Design review of the part built by this model. Coordinates are the model's own, in mm. A direction names the side the tool comes from. Coordinates: 2 decimals unless noted, no trailing zeros. Write each loop counter-clockwise with the first axis right and the second up, starting at its lowest first coordinate (ties: lowest second). Pieces come first, ordered by that corner, then holes. Notation, with made-up numbers: M 33.25,24 L 74.25,24 A26 cw 74.25,46 Z; hole C 19.5,63 d2. An arc over 180 degrees is marked long. Write each question's results on one line, items separated by ' | '. Start each with the question number.
```python
from build123d import *

# Parameters (mm, degrees)
F0_R     = 1.5
F1_DEPTH = 4


with BuildPart() as f1:
    # F0 (on Top) → F1 (new body)
    with BuildSketch(Plane.XY):
        with BuildLine():
            Line((10, 68.838424), (-25, 68.838424))
            Line((-25, 68.838424), (-25, 56.048434))
            Line((-25, 56.048434), (-15.945247, 35.027615))
            ThreePointArc((-15.945247, 35.027615), (-34.796929, 16.442581), (-37.185223, -9.921893))
            Line((-37.185223, -9.921893), (-47.426407, -15.834643))
            Line((-47.426407, -15.834643), (-56.234754, -20.920145))
            Line((-56.234754, -20.920145), (-64.615824, -25.758958))
            Line((-64.615824, -25.758958), (-47.115824, -56.069847))
            Line((-47.115824, -56.069847), (-36.039368, -49.674852))
            Line((-36.039368, -49.674852), (-29.243596, -40.556283))
            Line((-29.243596, -40.556283), (-22.362181, -31.322797))
            ThreePointArc((-22.362181, -31.322797), (3.158772, -38.356315), (27.185223, -27.242401))
            Line((27.185223, -27.242401), (37.426407, -33.155151))
            Line((37.426407, -33.155151), (46.234754, -38.240653))
            Line((46.234754, -38.240653), (54.615824, -43.079466))
            Line((54.615824, -43.079466), (72.115824, -12.768577))
            Line((72.115824, -12.768577), (61.039368, -6.373582))
            Line((61.039368, -6.373582), (49.744569, -5.047556))
            Line((49.744569, -5.047556), (38.307428, -3.704819))
            ThreePointArc((38.307428, -3.704819), (31.638157, 21.913734), (10, 37.164294))
            Line((10, 37.164294), (10, 59.160798))
            Line((10, 59.160798), (10, 68.838424))
        make_face()
        with Locations((-45.651723, -50.605746)):
            Circle(F0_R, mode=Mode.SUBTRACT)
        with Locations((-54.151723, -35.883314)):
            Circle(F0_R, mode=Mode.SUBTRACT)
        with Locations((-14.314554, -12.883314)):
            Circle(F0_R, mode=Mode.SUBTRACT)
        with Locations((58.151723, -28.955111)):
            Circle(F0_R, mode=Mode.SUBTRACT)
        with Locations((18.314554, -5.955111)):
            Circle(F0_R, mode=Mode.SUBTRACT)
        with Locations((66.651723, -14.232679)):
            Circle(F0_R, mode=Mode.SUBTRACT)
        with Locations((-4, 18.838424)):
            Circle(F0_R, mode=Mode.SUBTRACT)
        with Locations((-21, 64.838424)):
            Circle(F0_R, mode=Mode.SUBTRACT)
        with Locations((-4, 64.838424)):
            Circle(F0_R, mode=Mode.SUBTRACT)
    extrude(amount=F1_DEPTH)


solid = f1.part
```
Item 1: For faces 5 (the flat face through (-25, 63, 2)), 6 (the cylindrical face through (-12.93, -13.46, 1.97)), list the 3-axis set-ups (+Z, -Z, +X, -X, +Y, -Y) from which the entire face can be reached by the end or side of a thin tool; tool diameter is ignored.
Item 2: Draft analysis for pull direction X (two halves, no side actions). For faces 1 (the flat face through (3, -7, 0)), 2 (the cylindrical face through (58.96, -27.69, 1.97)), 3 (the flat face through (-20.54, 45.69, 1.97)), 4 (the flat face through (10, 53, 2)), state which applies: released by +X, released by -X, zero draft, split by the parting line, or undercut.
Item 3: We need section B-B on x = -4. State the section outline as (y, z) points, then the cut area to 3 significant figures.
Item 4: Wall thickness on L1, parallel to Y at x = -4, z = 2.8; L2, parallel to Y at x = -4.5, z = 0.5; L3, parallel to X at y = -50, z = 2.2: over which ranges is each line inside the solid? List them lowest first.
Item 5: We need section C-C on x = 44.5. State the section outline as (y, z) points, then the cut area to 3 significant figures.
Item 6: Insertion check: pin 1 Ø2 at (y, z) = (60, 2) entering from -X; pin 2 Ø1.5 at (y, z) = (-31, 0.5) entering from +X; pin 3 Ø2 at (y, z) = (-42, 3.5) entering from +X. Each pin has a flat end and moves straight along its axis. Give the tip position at first contact, or say it passes through.
Item 7: We need section A-A on z = 1. Count the separate pieces of the cut face and the enclosed holes in it, then the cut area to 3 significant figures.
Answer:
1) face 5: +Z, -Z, -X, +Y | face 6: +Z, -Z
2) face 1: zero draft | face 2: undercut | face 3: released by -X | face 4: released by +X
3) outline: M -38.28,0 L 17.34,0 L 17.34,4 L -38.28,4 Z; M 20.34,0 L 63.34,0 L 63.34,4 L 20.34,4 Z; M 66.34,0 L 68.84,0 L 68.84,4 L 66.34,4 Z | area: 404 mm^2
4) L1: y = -38.28 to 17.34, 20.34 to 63.34, 66.34 to 68.84 | L2: y = -38.22 to 17.42, 20.25 to 63.42, 66.25 to 68.84 | L3: x = -50.62 to -47.02, -44.28 to -36.6
5) outline: M -37.24,0 L -4.43,0 L -4.43,4 L -37.24,4 Z | area: 131 mm^2
6) pin 1: stops at x = -25 | pin 2: stops at x = 62.02 | pin 3: stops at x = 55.82
7) separate pieces: 1 | enclosed holes: 9 | area: 7,650 mm^2
